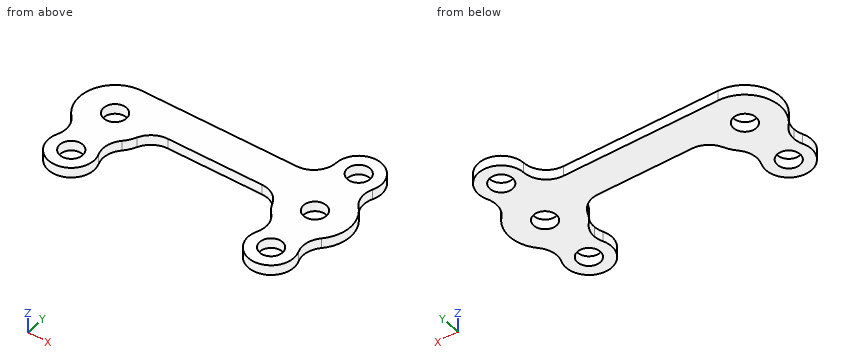
from build123d import *

# Parameters (mm, degrees)
SKETCH1_R           = 1.7859375
SKETCH1_R_2         = 3.571875
BOSS_EXTRUDE1_DEPTH = 1.5875
FILLET1_R           = 3.571875


with BuildPart() as part:
    # Sketch1 → Boss-Extrude1 (new body)
    # profile 1 of 10: a face of its own
    with BuildSketch(Plane.XY):
        with BuildLine():
            Line((5.55625, 0), (26.19375, 0))
            ThreePointArc((26.19375, 0), (27.821137947, -3.928862053), (31.75, -5.55625))
            ThreePointArc((31.75, -5.55625), (37.30625, 0), (31.75, 5.55625))
            Line((31.75, 5.55625), (0, 5.55625))
            ThreePointArc((0, 5.55625), (-5.55625, 0), (0, -5.55625))
            ThreePointArc((0, -5.55625), (3.928862053, -3.928862053), (5.55625, 0))
        make_face()
        Circle(SKETCH1_R, mode=Mode.SUBTRACT)
        with Locations((31.75, 0)):
            Circle(SKETCH1_R, mode=Mode.SUBTRACT)
    # profile 2 of 10: a face of its own
    with BuildSketch(Plane.XY):
        with Locations((0, -9.128125)):
            Circle(SKETCH1_R_2)
        with Locations((0, -9.128125)):
            Circle(SKETCH1_R, mode=Mode.SUBTRACT)
    # profile 3 of 10: a face of its own
    with BuildSketch(Plane.XY):
        with Locations((31.75, -9.128125)):
            Circle(SKETCH1_R_2)
        with Locations((31.75, -9.128125)):
            Circle(SKETCH1_R, mode=Mode.SUBTRACT)
    # profile 4 of 10: a face of its own
    with BuildSketch(Plane.XY):
        with Locations((31.75, 9.128125)):
            Circle(SKETCH1_R_2)
        with Locations((31.75, 9.128125)):
            Circle(SKETCH1_R, mode=Mode.SUBTRACT)
    # profile 5 of 10: a face of its own
    with BuildSketch(Plane.XY):
        with BuildLine():
            ThreePointArc((28.178125, 9.128125), (27.131947034, 6.602427966), (24.60625, 5.55625))
            Line((24.60625, 5.55625), (31.75, 5.55625))
            ThreePointArc((31.75, 5.55625), (29.224302966, 6.602427966), (28.178125, 9.128125))
        make_face()
    # profile 6 of 10: a face of its own
    with BuildSketch(Plane.XY):
        with BuildLine():
            ThreePointArc((31.75, 5.55625), (33.924184828, 5.113201971), (35.751636409, 3.854714012))
            ThreePointArc((35.751636409, 3.854714012), (34.811446668, 5.68510327), (35.037058415, 7.730434766))
            ThreePointArc((35.037058415, 7.730434766), (33.720522292, 6.148975304), (31.75, 5.55625))
        make_face()
    # profile 7 of 10: a face of its own
    with BuildSketch(Plane.XY):
        with BuildLine():
            ThreePointArc((35.751636291, -3.854714135), (33.92418475, -5.113202004), (31.75, -5.55625))
            ThreePointArc((31.75, -5.55625), (33.720522308, -6.148975314), (35.037058429, -7.730434799))
            ThreePointArc((35.037058429, -7.730434799), (34.811446649, -5.685103372), (35.751636291, -3.854714135))
        make_face()
    # profile 8 of 10: a face of its own
    with BuildSketch(Plane.XY):
        with BuildLine():
            ThreePointArc((31.75, -5.55625), (29.575815225, -5.113201993), (27.748363671, -3.854714095))
            ThreePointArc((27.748363671, -3.854714095), (28.48850069, -4.996759503), (28.747758155, -6.332744565))
            ThreePointArc((28.747758155, -6.332744565), (28.675829783, -7.045951842), (28.462941571, -7.730434799))
            ThreePointArc((28.462941571, -7.730434799), (29.779477692, -6.148975314), (31.75, -5.55625))
        make_face()
    # profile 9 of 10: a face of its own
    with BuildSketch(Plane.XY):
        with BuildLine():
            ThreePointArc((3.287058481, -7.730434921), (3.061446618, -5.685103543), (4.001636142, -3.854714289))
            ThreePointArc((4.001636142, -3.854714289), (2.174184651, -5.113202046), (0, -5.55625))
            ThreePointArc((0, -5.55625), (1.970522363, -6.148975351), (3.287058481, -7.730434921))
        make_face()
    # profile 10 of 10: a face of its own
    with BuildSketch(Plane.XY):
        with BuildLine():
            ThreePointArc((-3.287058429, -7.730434799), (-1.970522308, -6.148975314), (0, -5.55625))
            ThreePointArc((0, -5.55625), (-2.174184798, -5.113201984), (-4.001636364, -3.854714059))
            ThreePointArc((-4.001636364, -3.854714059), (-3.26149932, -4.99675948), (-3.002241845, -6.332744565))
            ThreePointArc((-3.002241845, -6.332744565), (-3.074170217, -7.045951842), (-3.287058429, -7.730434799))
        make_face()
    extrude(amount=BOSS_EXTRUDE1_DEPTH)

    # Fillet1
    fillet1_edges = [part.edges().sort_by_distance(p)[0] for p in [
        (26.19375, 0, 0.79375),
        (5.55625, 0, 0.79375),
    ]]
    fillet(fillet1_edges, radius=FILLET1_R)


solid = part.part
The listing builds one solid part. Answer for the finished solid, in the listing's coordinates (mm). Round coordinates to 2 decimals unless told otherwise and drop trailing zeros. Loops run counter-clockwise (first coordinate to the right, second up) from the corner with the lowest first, then second, coordinate; pieces in that order, holes last. Notation, with made-up numbers: M 63.25,70.5 L 104.25,70.5 A28 ccw 104.25,96.5 Z; hole C 83.25,-2.75 d9. An arc over 180 degrees is marked long. Write each question's results on one line, items separated by ' | '. Start each with the question number.
1) Each of these flat-tipped pins is pushed along its axis until it touches: pin 1 (4.5 mm diameter, centred on x = 0, y = -9.13, fed in from +Z); pin 2 (0.5 mm diameter, centred on x = 12.5, z = 0.5, fed in from +Y); pin 3 (3 mm diameter, centred on x = 31.75, y = -9.13, fed in from +Z). Where does it stop, or does it pass through?
2) Find section B-B on y = 10.5. Write down the section's boundary in (x, z).
3) Straight lines are drawn through the part: probe 1 along Y at (x, z) = (31.75, 1.05); probe 2 along Y at (x, z) = (0, 0.75); probe 3 along X at (y, z) = (-8.5, 0.8). For each, find the intervals that lie inside material, in ascending order.
4) Find section A-A on x = 31.75. Write down the section's boundary in (y, z).
5) Find section C-C on z = 0.7. Write down the section's boundary in (x, y), plus the area to 3 significant figures.
6) Find section D-D on y = 0.5. Write down the section's boundary in (x, z).
Final values:
1) pin 1: z = 1.59 | pin 2: y = 5.56 | pin 3: through
2) outline: M 28.45,0 L 30.61,0 L 30.61,1.59 L 28.45,1.59 Z; M 32.89,0 L 35.05,0 L 35.05,1.59 L 32.89,1.59 Z
3) probe 1: -12.7 to -10.91, -7.34 to -1.79, 1.79 to 7.34, 10.91 to 12.7 | probe 2: -12.7 to -10.91, -7.34 to -1.79, 1.79 to 5.56 | probe 3: -3.52 to -1.67, 1.67 to 3.52, 28.23 to 30.08, 33.42 to 35.27
4) outline: M -12.7,0 L -10.91,0 L -10.91,1.59 L -12.7,1.59 Z; M -7.34,0 L -1.79,0 L -1.79,1.59 L -7.34,1.59 Z; M 1.79,0 L 7.34,0 L 7.34,1.59 L 1.79,1.59 Z; M 10.91,0 L 12.7,0 L 12.7,1.59 L 10.91,1.59 Z
5) outline: M -4,-3.85 A3.57 cw -3.29,-7.73 A3.57 ccw long 3.29,-7.73 A3.57 cw 4,-3.85 A5.56 ccw 5.11,-2.17 A3.57 cw 8.4,0 L 23.35,0 A3.57 cw 26.64,-2.17 A5.56 ccw 27.75,-3.85 A3.57 cw 28.46,-7.73 A3.57 ccw long 35.04,-7.73 A3.57 cw 35.75,-3.85 A5.56 ccw 35.75,3.85 A3.57 cw 35.04,7.73 A3.57 ccw long 28.18,9.13 A3.57 cw 24.61,5.56 L 0,5.56 A5.56 ccw Z; hole C 0,-9.13 d3.57; hole C 0,0 d3.57; hole C 31.75,-9.13 d3.57; hole C 31.75,0 d3.57; hole C 31.75,9.13 d3.57 | area: 414 mm²
6) outline: M -5.53,0 L -1.71,0 L -1.71,1.59 L -5.53,1.59 Z; M 1.71,0 L 30.04,0 L 30.04,1.59 L 1.71,1.59 Z; M 33.46,0 L 37.28,0 L 37.28,1.59 L 33.46,1.59 Z
